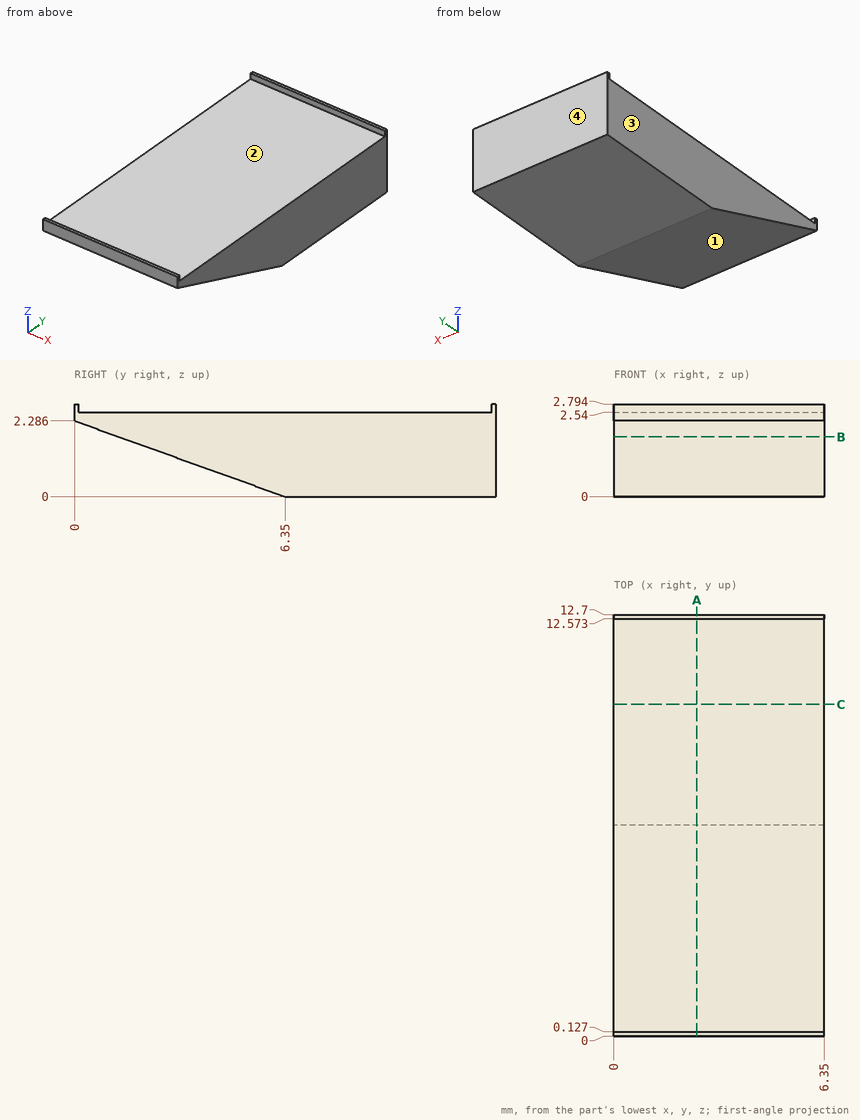
Can you work these out from the drawing? Everything is in mm from the part's minimum corner. Round coordinates to 2 decimals unless told otherwise and drop trailing zeros. Loops run counter-clockwise (first coordinate to the right, second up) from the corner with the lowest first, then second, coordinate; pieces in that order, holes last. Notation, with made-up numbers: (79, -12) - (133, -12) arc R23 ccw to (133, 0) - close; hole circle Ø3 at (70.25, -5). An arc over 180 degrees is marked (long way). One line per question, with ' | ' between items. Start each with the question number.
Q1. I want a section at C-C (y = 10). Write out the boundary of the cut face in (x, z), then the cut area to 3 significant figures.
Q2. I want a section at A-A (x = 2.5). Write out the boundary of the cut face in (y, z), then the cut area to 3 significant figures.
Q3. Please list where these lines run through material, in increasing order: line 1 (Z direction, x = 3.5, y = 8.25); line 2 (Z direction, x = 2.75, y = 6). Write a range as [from, to].
Q4. We'd pull the mould along Y, two halves only. Please class the marked faces 1, 2, 3 and 4: +Y half, -Y half, draft (parallel to the pull), parting line (faces both ways), or undercut.
Q5. I want a section at B-B (z = 1.8). Write out the boundary of the cut face in (x, y), then the cut area to 3 significant figures.
Q6. Will this pin go through, and if not, where does the flat tip stop? pin 1 (1 mm diameter, centred on x = 3, y = 4, fed in from -Z).
Response values:
1) outline: (0, 0) - (6.35, 0) - (6.35, 2.54) - (0, 2.54) - close | area: 16.1 mm²
2) outline: (0, 2.29) - (6.35, 0) - (12.7, 0) - (12.7, 2.79) - (12.57, 2.79) - (12.57, 2.54) - (0.13, 2.54) - (0.13, 2.79) - (0, 2.79) - close | area: 25.1 mm²
3) line 1: z = [0, 2.54] | line 2: z = [0.13, 2.54]
4) face 1: -Y half | face 2: undercut | face 3: draft | face 4: +Y half
5) outline: (0, 1.35) - (6.35, 1.35) - (6.35, 12.7) - (0, 12.7) - close | area: 72.1 mm²
6) pin 1: stops at z = 0.67
